Can you work these out from the model? Positions are in its coordinate system, mm. A direction names the side the tool comes from. Round coordinates to 2 decimals unless told otherwise and drop trailing zeros. Loops run counter-clockwise (first coordinate to the right, second up) from the corner with the lowest first, then second, coordinate; pieces in that order, holes last. Notation, with made-up numbers: (68.5, 33) -> (113.5, 33) arc R10 ccw to (113.5, 46) -> close; hole circle Ø2 at (-8.5, 34.5). An arc over 180 degrees is marked (long way). Write item = value, one per line.
from build123d import *

# Parameters (mm, degrees)
F0_W     = 38
F0_H     = 10
F1_DEPTH = 5
F2_R     = 1.5
F3_DEPTH = 5
F4_W     = 8
F4_H     = 5
F5_DEPTH = 5
F6_R     = 1.5
F7_DEPTH = 5
F8_R     = 4.99999


# Not quite as in the source:
# - a fillet or chamfer is up to 0.001 mm smaller than in the source, because OpenCascade refuses the exact size
# - a feature names something its author has since deleted; it is built from what else it names


with BuildPart() as f1:
    # F0 (on Top) → F1 (new body)
    with BuildSketch(Plane.XY):
        Polygon((20, -50), (20, 50), (-20, 50), (-20, 40), (-20, 12), (-20, 10), (-20, -50), align=None)
        with Locations((-39, 45)):
            Rectangle(F0_W, F0_H)
        Polygon((-58, 40), (-58, 50), (-60, 50), (-60, 10), (-20, 10), (-20, 12), (-58, 12), align=None)
    extrude(amount=F1_DEPTH)

    # F2 (on face) → F3 (cut)
    with BuildSketch(Plane.XY.offset(5)):
        with Locations((-35, 42)):
            Circle(F2_R)
        with Locations((-5, 15.5)):
            Circle(F2_R)
    extrude(amount=-F3_DEPTH, mode=Mode.SUBTRACT)

    # F4 (on face) → F5 (join)
    with BuildSketch(Plane(origin=(0, 0, 0), x_dir=(1, 0, 0), z_dir=(0, 0, -1))):
        with Locations((16, -47.5)):
            Rectangle(F4_W, F4_H)
        with Locations((-56, -47.5)):
            Rectangle(F4_W, F4_H)
    extrude(amount=F5_DEPTH)

    # F6 (on face) → F7 (cut)
    with BuildSketch(Plane(origin=(0, 50, 0), x_dir=(-1, 0, 0), z_dir=(0, 1, 0))):
        with BuildLine():
            ThreePointArc((-14.5, -2.5), (-16, -1), (-17.5, -2.5))
            ThreePointArc((-17.5, -2.5), (-16, -4), (-14.5, -2.5))
        make_face()
        with Locations((56, -2.5)):
            Circle(F6_R)
    extrude(amount=-F7_DEPTH, mode=Mode.SUBTRACT)

    # F8 (radius 5 in the source; OpenCascade refuses exactly that, so slightly less here)
    f8_edges = [f1.edges().sort_by_distance(p)[0] for p in [
        (20, -2.5, 0),
        (-20, 26, 0),
        (-20, -20, 0),
        (20, -50, 2.5),
        (0, -50, 0),
        (-20, -50, 2.5),
        (-58, 12, 2.5),
        (-60, 10, 2.5),
    ]]
    fillet(f8_edges, radius=F8_R)


solid = f1.part
1. Suppose I cut it at A-A, the plane x = -28. List the corners of the cut face in (y, z) for me, and give its area (3 significant figures).
Entries:
outline = (10, 0) -> (12, 0) -> (12, 5) -> (10, 5) -> close; (40, 0) -> (50, 0) -> (50, 5) -> (40, 5) -> close
area = 60.0 mm²
2. Suppose I cut it at D-D, the plane z = 2. List the corners of the cut face in (x, y) for me.
Entries:
outline = (-60, 15) arc R5 ccw to (-55, 10) -> (-19, 10) -> (-19, -45) arc R4 ccw to (-15, -49) -> (15, -49) arc R4 ccw to (19, -45) -> (19, 45) -> (20, 45) -> (20, 50) -> (-60, 50) -> close; hole (-58, 17) arc R5 ccw to (-53, 12) -> (-19, 12) -> (-19, 40) -> (-58, 40) -> close; hole circle Ø3 at (-35, 42); hole circle Ø3 at (-5, 15.5)
3. I'm going to push flat-ended pins straight in: pin 1 (2 mm diameter, centred on y = -34.5, z = 0.5, fed in from +X); pin 2 (6 mm diameter, centred on y = -19.5, z = 3, fed in from -X); pin 3 (2.5 mm diameter, centred on y = 30.5, z = 1.5, fed in from +X). Where does each tip first touch, or does it pass through?
Entries:
pin_1 = 18.57
pin_2 = -20
pin_3 = 19.47
4. Suppose I cut it at B-B, the plane z = -2.5. List the corners of the cut face in (x, y) for me, and give its area (3 significant figures).
Entries:
outline = (-60, 45) -> (-57.5, 45) -> (-57.5, 50) -> (-60, 50) -> close; (-54.5, 45) -> (-52, 45) -> (-52, 50) -> (-54.5, 50) -> close; (12, 45) -> (14.5, 45) -> (14.5, 50) -> (12, 50) -> close; (17.5, 45) -> (20, 45) -> (20, 50) -> (17.5, 50) -> close
area = 50.0 mm²
5. We'd pull the mould along Y, two halves only. Please class faces 1 (the cylindrical face through (14.5, 47.54, -2.57)), 2 (the flat face through (-21, 50, 2)), 3 (the flat face through (-37, 40, 2)), 4 (the cylindrical face through (-59, 12, 3)): released by +Y, released by -Y, zero draft, split by the parting line, or undercut.
Entries:
face_1 = zero draft
face_2 = released by +Y
face_3 = undercut
face_4 = released by -Y
6. For faces 5 (the cylindrical face through (-57, 14, 3)), 6 (the cylindrical face through (-18, 26, 1)), 7 (the flat face through (12, 48, -2)), 8 (the cylindrical face through (18, 1, 1)), which set-ups out of +Z, -Z, +X, -X, +Y, -Y let a thin tool reach every point of the face, with its end or its side?
Entries:
face_5 = +Z, -Z
face_6 = -Z
face_7 = -Z, +Y, -Y
face_8 = -Z, +X, -Y
7. I need wall thicknesses on line 1 (Y direction, x = -35, z = 2.75); line 2 (Y direction, x = -43.5, z = 2.75); line 3 (Z direction, x = -56, y = 47.65). Which ranges of each line are inside material? Lowest first, please. Write a range as [from, to].
Entries:
line_1 = [10, 12], [40, 40.5], [43.5, 50]
line_2 = [10, 12], [40, 50]
line_3 = [-5, -4], [-1, 5]
